Input: part model. Units: mm. Frame: model coordinates. Face numbers are marked on the shaded views. Round coordinates to 2 decimals unless told otherwise and drop trailing zeros. Order: outer loops, then holes, each group sorted by start corner. A loop starts at its lowest first (then second) coordinate and runs counter-clockwise, first axis right, second up. Notation, with made-up numbers: (56.25, 69) - (110.25, 69) arc R12 ccw to (110.25, 90) - close; hole circle Ø8 at (67, -18). An arc over 180 degrees is marked (long way). One line per item, written item: value. Start each with the question number.
Autodesk Inventor part; units mm, degrees
ref_plane "YZ Plane" through (0, 0, 0) normal (1, 0, 0) x (0, 1, 0)
ref_plane "XZ Plane" through (0, 0, 0) normal (0, 1, 0) x (-1, 0, 0)
ref_plane "XY Plane" through (0, 0, 0) normal (0, 0, 1) x (1, 0, 0)
sketch "Sketch1" plane through (0, 0, 0) normal (0, 0, 1) x (1, 0, 0)
  circle A0 centre (0, 15) radius 12.5
  arc A1 (15, 15) -> (-15, 15) centre (0, 15) ccw
  line L0 (-15, 15) -> (-15, 0)
  line L1 (15, 15) -> (15, 0)
  line L2 (15, 0) -> (-15, 0)
  point P0 (0, 0)
  dimension "d0" = 25
  dimension "d1" = 30
  dimension "d2" = 15
extrude "Extrusion1" add sketch "Sketch1" along normal blind 50
sketch "Sketch2" plane through (0, 0, 50) normal (0, 0, 1) x (1, 0, 0)
  circle A0 centre (0, 15) radius 12.5 construction
  line L0 (0, 27.5) -> (0, 2.5) construction
  circle A1 centre (0, 15) radius 12.5
  point P0 (0, 0)
extrude "Extrusion2" add sketch "Sketch2" against normal blind 2
sketch "Sketch3" plane through (0, 0, 50) normal (0, 0, 1) x (1, 0, 0)
  circle A0 centre (0, 15) radius 12.5 construction
  line L0 (0, 2.5) -> (0, 27.5) construction
  circle A1 centre (0, 23.5) radius 1
  circle A2 centre (0, 6.5) radius 1
  circle A3 centre (0, 15) radius 3.75
  point P0 (0, 0)
  dimension "d7" = 2
  dimension "d8" = 2
  dimension "d9" = 8.5
  dimension "d10" = 17
  dimension "d11" = 7.5
extrude "Extrusion3" cut sketch "Sketch3" against normal blind 2.5
thread "Thread1"
thread "Thread2"
properties part number "bancada"
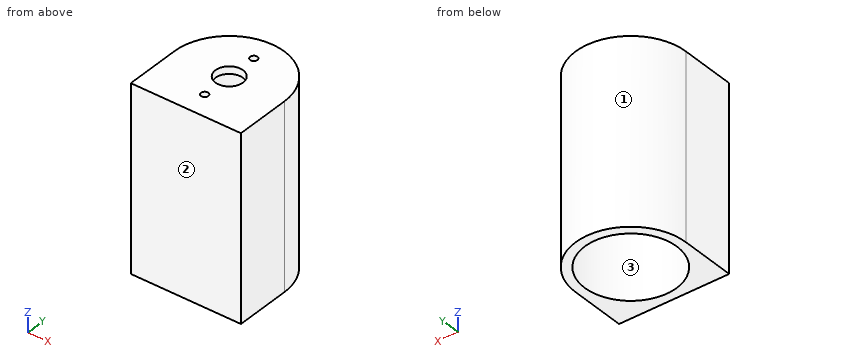
1. Section D-D (y = 3.5). Return the cut outline in (x, z).
2. Pull-direction query (X, two-part tool) for the marked faces 1, 2 and 3; classes: released by +X, released by -X, zero draft, split by the parting line, or undercut.
3. Pin query (flat end, axial travel): pin 1 (1.5 mm diameter, centred on x = -6.5, z = 17.5, fed in from +Y); pin 2 (1.5 mm diameter, centred on x = 2, z = 17.5, fed in from +Y); pin 3 (10 mm diameter, centred on x = 9, z = 32.5, fed in from +Y). Return the tip coordinate at first contact, or that it passes through.
4. Line query: line 1 (Y direction, x = 0, z = 49.45); line 2 (Y direction, x = 0, z = 21.5); line 3 (Z direction, x = -4.25, y = 19.25). Output: solid intervals per line, ascending. Write a range as from..to.
5. Section B-B (y = 12.5). Return the cut outline in (x, z), then the cut area to 3 significant figures.
6. Section A-A (x = 0). Return the cut outline in (y, z).
7. Section C-C (z = 12.5). Return the cut outline in (x, y).
Solved:
1. outline: (-15, 0) - (-4.9, 0) - (-4.9, 48) - (4.9, 48) - (4.9, 0) - (15, 0) - (15, 50) - (-15, 50) - close
2. face 1: split by the parting line
2. face 2: zero draft
2. face 3: undercut
3. pin 1: stops at y = 28.85
3. pin 2: stops at y = 29.95
3. pin 3: stops at y = 29.46
4. line 1: y = 0..5.5, 7.5..11.25, 18.75..22.5, 24.5..30
4. line 2: y = 0..2.5, 27.5..30
4. line 3: z = 48..50
5. outline: (-15, 0) - (-12.25, 0) - (-12.25, 48) - (-2.8, 48) - (-2.8, 50) - (-15, 50) - close; (2.8, 48) - (12.25, 48) - (12.25, 0) - (15, 0) - (15, 50) - (2.8, 50) - close
5. area: 313 mm²
6. outline: (0, 0) - (2.5, 0) - (2.5, 48) - (5.5, 48) - (5.5, 50) - (0, 50) - close; (7.5, 48) - (11.25, 48) - (11.25, 50) - (7.5, 50) - close; (18.75, 48) - (22.5, 48) - (22.5, 50) - (18.75, 50) - close; (24.5, 48) - (27.5, 48) - (27.5, 0) - (30, 0) - (30, 50) - (24.5, 50) - close
7. outline: (-15, 0) - (15, 0) - (15, 15) arc R15 ccw to (-15, 15) - close; hole circle Ø25 at (0, 15)
